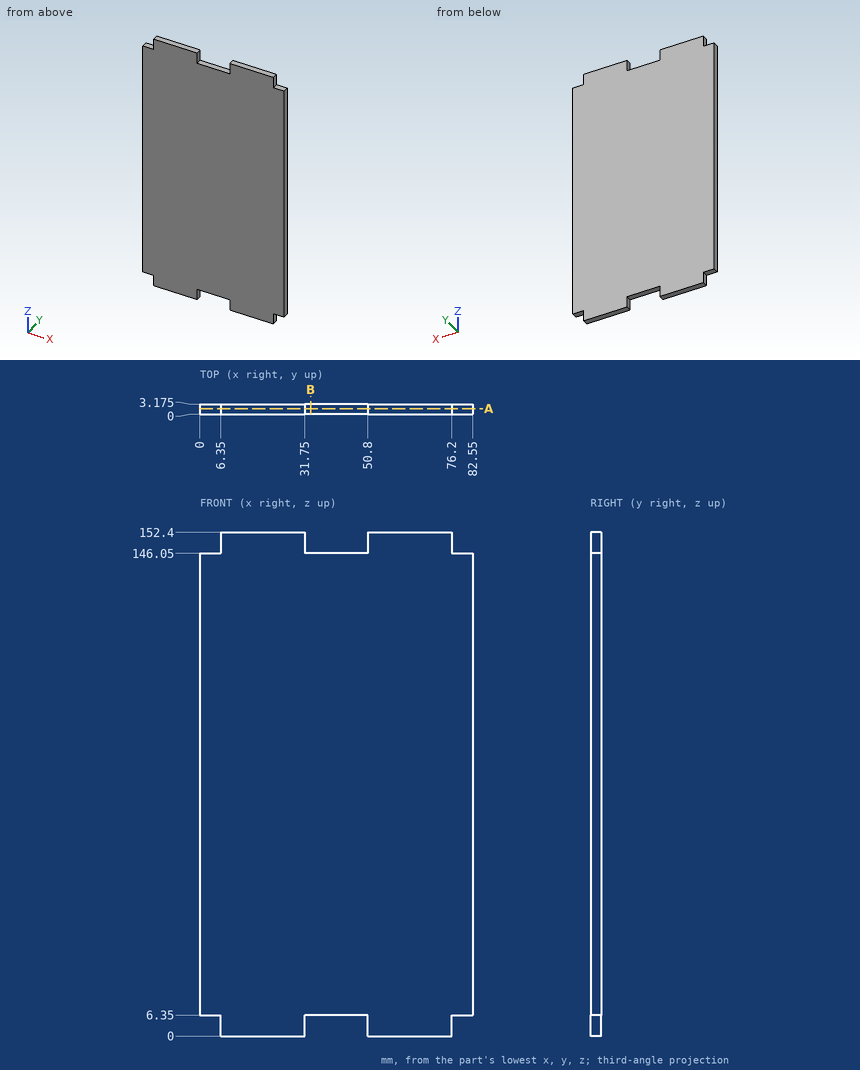
Part print with two shaded views. Sizes in mm from the minimum x, y, z corner. Coordinates: 2 decimals unless noted, no trailing zeros. Write each loop counter-clockwise with the first axis right and the second up, starting at its lowest first coordinate (ties: lowest second). Pieces come first, ordered by that corner, then holes. Notation, with made-up numbers: (8.25, 28.5) - (12.25, 28.5) arc R7 cw to (12.25, 37.5) - close; hole circle Ø6 at (12.25, 22). An arc over 180 degrees is marked (long way). Use a Markdown table: item, result. Add a question column.
Item 1: Band-saw the part on A-A, the plane y = 1.75. Write the cut outline in (x, z), and give its area (3 significant figures).
Item 2: Drill centre line: line 1 along Z through (x, y) = (77, 1.75). Where is it in solid material? Low to high.
Item 3: Band-saw the part on B-B, the plane x = 33.5. Write the cut outline in (y, z) (3 decimals), and give its area (3 significant figures).
Item 4: Drop flat-ended pins along their axis: pin 1 (1.6 mm diameter, centred on x = 2, y = 1.5, fed in from -Z); pin 2 (1 mm diameter, centred on x = 41, y = 1.5, fed in from +Z); pin 3 (1.6 mm diameter, centred on y = 1.5, z = 4.5, fed in from +X). Give the stop position or say it passes through.
A:
| question | item | result |
|---|---|---|
| 1 | outline | (0, 6.35) - (6.35, 6.35) - (6.35, 0) - (31.75, 0) - (31.75, 6.35) - (50.8, 6.35) - (50.8, 0) - (76.2, 0) - (76.2, 6.35) - (82.55, 6.35) - (82.55, 146.05) - (76.2, 146.05) - (76.2, 152.4) - (50.8, 152.4) - (50.8, 146.05) - (31.75, 146.05) - (31.75, 152.4) - (6.35, 152.4) - (6.35, 146.05) - (0, 146.05) - close |
| 1 | area | 12,200 mm² |
| 2 | line 1 | z = 6.35 to 146.05 |
| 3 | outline | (0, 6.35) - (3.175, 6.35) - (3.175, 146.05) - (0, 146.05) - close |
| 3 | area | 444 mm² |
| 4 | pin 1 | stops at z = 6.35 |
| 4 | pin 2 | stops at z = 146.05 |
| 4 | pin 3 | stops at x = 76.2 |
